Build history of the part. All positions in model axes, mm. Face numbers are marked on the shaded views. A direction names the side the tool comes from. Give positions to 0.01 mm unless a question says otherwise; leave off trailing zeros. Order: outer loops, then holes, each group sorted by start corner. A loop starts at its lowest first (then second) coordinate and runs counter-clockwise, first axis right, second up. Notation, with made-up numbers: M 81.25,75.5 L 125.25,75.5 A25 ccw 125.25,96.5 Z; hole C 36,3 d6. An arc over 180 degrees is marked long. One line per item, written item: value. Start each with the question number.
from build123d import *

# Parameters (mm, degrees)
SKETCH044_R     = 1.6
PAD025_DEPTH    = 9
FILLET013_R     = 1
CHAMFER007_SIZE = 0.4


with BuildPart() as part:
    # Sketch044 → Pad025 (new body)
    with BuildSketch(Plane.YZ):
        Polygon((-10, 17), (13, 17), (13, -37), (-10, -37), (-10, -30), (10, -30), (10, 10), (-10, 10), align=None)
        with Locations((-5, 14.5)):
            Circle(SKETCH044_R, mode=Mode.SUBTRACT)
        with Locations((5, 14.5)):
            Circle(SKETCH044_R, mode=Mode.SUBTRACT)
        with Locations((-5, -34.5)):
            Circle(SKETCH044_R, mode=Mode.SUBTRACT)
        with Locations((5, -34.5)):
            Circle(SKETCH044_R, mode=Mode.SUBTRACT)
    extrude(amount=-PAD025_DEPTH)

    # Fillet013
    fillet013_edges = [part.edges().sort_by_distance(p)[0] for p in [
        (-4.5, -10, 17),
        (-4.5, -10, 10),
        (-4.5, -10, -30),
        (-4.5, -10, -37),
        (-4.5, 13, -37),
        (-4.5, 13, 17),
    ]]
    fillet(fillet013_edges, radius=FILLET013_R)

    # Chamfer007
    chamfer007_edges = [part.edges().sort_by_distance(p)[0] for p in [
        (0, 1.5, 17),
        (0, -9.707107, 16.707107),
        (0, 12.707107, 16.707107),
        (0, -10, 13.5),
        (0, 13, -10),
        (0, -9.707107, 10.292893),
        (0, 12.707107, -36.707107),
        (0, 0.5, 10),
        (0, 1.5, -37),
        (0, 10, -10),
        (0, -9.707107, -36.707107),
        (0, 0.5, -30),
        (0, -10, -33.5),
        (0, -9.707107, -30.292893),
        (0, -6.6, 14.5),
        (0, 3.4, 14.5),
        (0, -6.6, -34.5),
        (0, 3.4, -34.5),
        (-9, 1.5, 17),
        (-9, -9.707107, 16.707107),
        (-9, 12.707107, 16.707107),
        (-9, -10, 13.5),
        (-9, 13, -10),
        (-9, -9.707107, 10.292893),
        (-9, 12.707107, -36.707107),
        (-9, 0.5, 10),
        (-9, 1.5, -37),
        (-9, 10, -10),
        (-9, -9.707107, -36.707107),
        (-9, 0.5, -30),
        (-9, -10, -33.5),
        (-9, -9.707107, -30.292893),
        (-9, -6.6, 14.5),
        (-9, 3.4, 14.5),
        (-9, -6.6, -34.5),
        (-9, 3.4, -34.5),
    ]]
    chamfer(chamfer007_edges, length=CHAMFER007_SIZE)


with BuildPart() as part_1:
    # Body025 placement: moved
    add(part.part.moved(Location((-8, 0, 0))))


solid = part_1.part
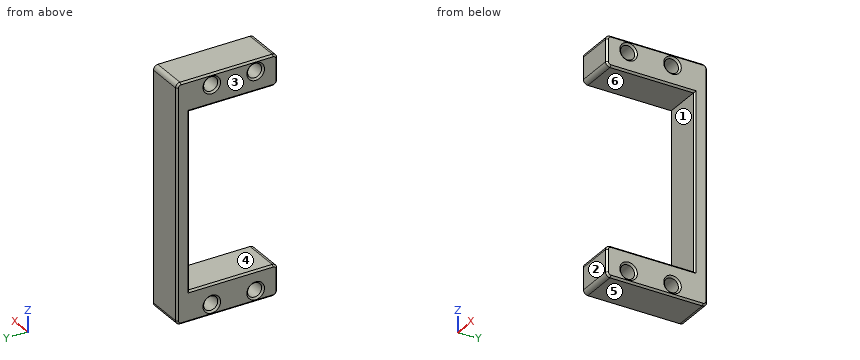
1) Drop flat-ended pins along their axis: P1, Ø5, axis at x = -12.5, z = -13, coming from the -Y side; P2, Ø3.5, axis at y = 5, z = -34.5, coming from the +X side; P3, Ø2.5, axis at y = 5, z = 14.5, coming from the +X side. Give the stop position or say it passes through.
2) Tool access for the marked faces 1 and 2: list every direction of +Z, -Z, +X, -X, +Y, -Y with a clear straight run to the whole face (end or side of a thin tool).
3) Slice it at D-D (z = -4.5). List the corners of the cut face in (x, y).
4) Slice it at B-B (z = -34.5). List the corners of the cut face in (x, y), plus the area to 3 significant figures.
5) Slice it at C-C (y = 5). State how many separate pieces and enclosed holes the cut face has, plus the area to 3 significant figures.
6) Slice it at A-A (x = -13.5). List the corners of the cut face in (y, z).
7) Drill centre lines: line 1 (Z direction, x = -11.5, y = -5); line 2 (Z direction, x = -9, y = -1.75); line 3 (Z direction, x = -16.5, y = 3.75). Where is each one in solid material? Low to high.
8) Pull direction Z, two halves, no side cores. Call the marked faces 3, 4, 5 and 6: pulls with the +Z half, pulls with the -Z half, needs draft (parallel to the pull), parting line crosses it, or undercut.
Results list:
1. P1: stops at y = 10
1. P2: stops at x = -8.25
1. P3: passes through
2. face 1: +X, -X, -Y
2. face 2: +Z, -Z, +X, -X, -Y
3. outline: M -17,10.4 L -16.6,10 L -8.4,10 L -8,10.4 L -8,12.6 L -8.4,13 L -16.6,13 L -17,12.6 Z
4. outline: M -17,-9.6 L -16.6,-10 L -8.4,-10 L -8,-9.6 L -8,-7 L -8.4,-6.6 L -16.6,-6.6 L -17,-7 Z; M -17,-3 L -16.6,-3.4 L -8.4,-3.4 L -8,-3 L -8,3 L -8.4,3.4 L -16.6,3.4 L -17,3 Z; M -17,7 L -16.6,6.6 L -8.4,6.6 L -8,7 L -8,12.6 L -8.4,13 L -16.6,13 L -17,12.6 Z
4. area: 148 mm²
5. separate pieces: 4
5. enclosed holes: 0
5. area: 67.1 mm²
6. outline: M -10,-36 A1 ccw -9,-37 L 12,-37 A1 ccw 13,-36 L 13,16 A1 ccw 12,17 L -9,17 A1 ccw -10,16 L -10,11 A1 ccw -9,10 L 10,10 L 10,-30 L -9,-30 A1 ccw -10,-31 Z; hole C -5,-34.5 d3.2; hole C -5,14.5 d3.2; hole C 5,-34.5 d3.2; hole C 5,14.5 d3.2
7. line 1: z = -37 to -36.1, -32.9 to -30, 10 to 12.9, 16.1 to 17
7. line 2: z = -37 to -30, 10 to 17
7. line 3: z = -37 to -35.5, -33.5 to -30, 10 to 13.5, 15.5 to 17
8. face 3: needs draft
8. face 4: undercut
8. face 5: pulls with the -Z half
8. face 6: undercut
